CAD build for the part. Positions are in the model's coordinates, mm. Face numbers are marked on the shaded views. A direction names the side the tool comes from. Give positions to 0.01 mm unless a question says otherwise; leave off trailing zeros. Loops run counter-clockwise (first coordinate to the right, second up) from the corner with the lowest first, then second, coordinate; pieces in that order, holes last.
Item 1: Which spindle directions (+Z, -Z, +X, -X, +Y, -Y) get a long thin tool onto all of the face, cutting with end or side? Do the marked faces 5, 6 and 7. Say none if no direction does.
Item 2: Probe probe 1 along Z at (x, y) = (13.5, 10); probe 2 along Y at (x, z) = (0, 13.75); probe 3 along Y at (x, z) = (-5, 4.5) (3 decimals). List the from-to ranges inside material, lowest first.
Item 3: Saw through at A-A on y = 0. Give the cut face in (x, z), plus the area to 3 significant figures.
Item 4: Mould opens along X. For the marked faces 1, 2, 3 and 4 say: released by +X, released by -X, zero draft, split by the parting line, or undercut.
Item 5: Saw through at C-C on z = 5.25. Give the cut face in (x, y).
Item 6: Drop flat-ended pins along their axis: P1, Ø1.5, axis at y = -2.5, z = 13, coming from the -X side; P2, Ø4.5, axis at x = -15, y = -7, coming from the +Z side; P3, Ø8, axis at y = 3.5, z = 4.5, coming from the +X side. Give the stop position or say it passes through.
Item 7: Saw through at B-B on x = 0. Give the cut face in (y, z).
Item 8: Saw through at D-D on y = -15. Give the cut face in (x, z), plus the area to 3 significant figures.
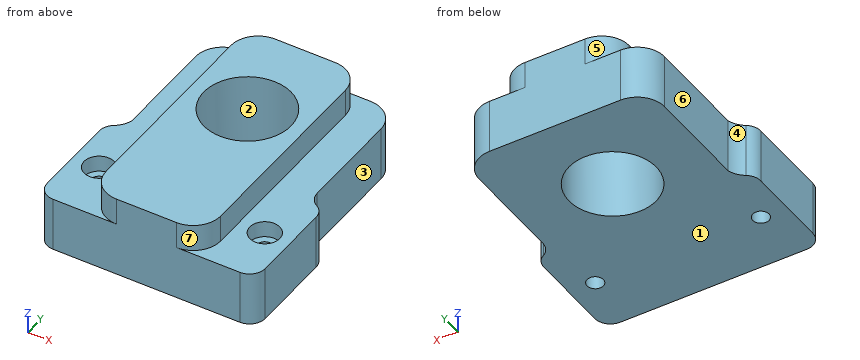
from build123d import *

# Parameters (mm, degrees)
F1_DEPTH  = 10
F3_DEPTH  = 5
F4_R      = 8
F5_DEPTH  = 25
F6_R      = 2.75
F6_R_2    = 1.5
F7_DEPTH  = 3
F8_DEPTH  = 25
F9_R      = 2.75
F9_R_2    = 1.5
F10_DEPTH = 3
F11_DEPTH = 25


with BuildPart() as f1:
    # F0 (on Top) → F1 (new body)
    with BuildSketch(Plane.XY):
        with BuildLine():
            Line((-17.1261427557, -29.75), (17.1261427557, -29.75))
            ThreePointArc((17.1261427557, -29.75), (19.1582667013, -28.9082667013), (20, -26.8761427557))
            Line((20, -26.8761427557), (20, -11.87280621))
            ThreePointArc((20, -11.87280621), (19.6060520694, -10.4205303214), (18.5322129268, -9.3664099655))
            ThreePointArc((18.5322129268, -9.3664099655), (17.4112395611, -8.2660209069), (17, -6.75))
            Line((17, -6.75), (17, 12))
            ThreePointArc((17, 12), (15.5355339059, 15.5355339059), (12, 17))
            Line((12, 17), (-12, 17))
            ThreePointArc((-12, 17), (-15.5355339059, 15.5355339059), (-17, 12))
            Line((-17, 12), (-17, -6.75))
            ThreePointArc((-17, -6.75), (-17.6456554571, -8.1178497679), (-18.730129695, -9.1722688421))
            ThreePointArc((-18.730129695, -9.1722688421), (-19.6627433299, -10.206041959), (-20, -11.5568613354))
            Line((-20, -11.5568613354), (-20, -26.8761427557))
            ThreePointArc((-20, -26.8761427557), (-19.1582667013, -28.9082667013), (-17.1261427557, -29.75))
        make_face()
    extrude(amount=F1_DEPTH)

    # F2 (on face) → F3 (join)
    with BuildSketch(Plane.XY.offset(10)):
        with BuildLine():
            Line((-10.5, 12), (-10.5, -24.75))
            ThreePointArc((-10.5, -24.75), (-9.0355339059, -28.2855339059), (-5.5, -29.75))
            Line((-5.5, -29.75), (5.5, -29.75))
            ThreePointArc((5.5, -29.75), (9.0355339059, -28.2855339059), (10.5, -24.75))
            Line((10.5, -24.75), (10.5, 12))
            ThreePointArc((10.5, 12), (9.0355339059, 15.5355339059), (5.5, 17))
            Line((5.5, 17), (-5.5, 17))
            ThreePointArc((-5.5, 17), (-9.0355339059, 15.5355339059), (-10.5, 12))
        make_face()
    extrude(amount=F3_DEPTH)

    # F4 (on face) → F5 (cut)
    with BuildSketch(Plane.XY.offset(15)):
        Circle(F4_R)
    extrude(amount=-F5_DEPTH, mode=Mode.SUBTRACT)

    # F6 (on face) → F7 (cut)
    with BuildSketch(Plane.XY.offset(10)):
        with Locations((-15.25, -19.2165020456)):
            Circle(F6_R)
        with Locations((-15.25, -19.2165020456)):
            Circle(F6_R_2, mode=Mode.SUBTRACT)
    extrude(amount=-F7_DEPTH, mode=Mode.SUBTRACT)

    # F8 (cut): a face of the model
    f8_faces = [f1.faces().sort_by_distance(p)[0] for p in [
        (-15.25, -19.2165020456, 10),
    ]]
    extrude(f8_faces, amount=-F8_DEPTH, mode=Mode.SUBTRACT)

    # F9 (on face) → F10 (cut)
    with BuildSketch(Plane.XY.offset(10)):
        with Locations((15.25, -19.3744744829)):
            Circle(F9_R)
        with Locations((15.25, -19.3744744829)):
            Circle(F9_R_2, mode=Mode.SUBTRACT)
    extrude(amount=-F10_DEPTH, mode=Mode.SUBTRACT)

    # F11 (cut): a face of the model
    f11_faces = [f1.faces().sort_by_distance(p)[0] for p in [
        (15.25, -19.3744744829, 10),
    ]]
    extrude(f11_faces, amount=-F11_DEPTH, mode=Mode.SUBTRACT)


solid = f1.part
Results below:
1. face 5: +Z, -X, +Y
1. face 6: +Z, -Z, -X, +Y
1. face 7: +Z, +X, -Y
2. probe 1: z = 0 to 10
2. probe 2: y = -29.75 to -8, 8 to 17
2. probe 3: y = -29.75 to -6.245, 6.245 to 17
3. outline: (-17, 0) - (-8, 0) - (-8, 15) - (-10.5, 15) - (-10.5, 10) - (-17, 10) - close; (8, 0) - (17, 0) - (17, 10) - (10.5, 10) - (10.5, 15) - (8, 15) - close
3. area: 205 mm2
4. face 1: zero draft
4. face 2: undercut
4. face 3: released by +X
4. face 4: released by -X
5. outline: (-20, -26.88) arc R2.87 ccw to (-17.13, -29.75) - (17.13, -29.75) arc R2.87 ccw to (20, -26.88) - (20, -11.87) arc R2.87 ccw to (18.53, -9.37) arc R3 cw to (17, -6.75) - (17, 12) arc R5 ccw to (12, 17) - (-12, 17) arc R5 ccw to (-17, 12) - (-17, -6.75) arc R4.24 cw to (-18.73, -9.17) arc R2.87 ccw to (-20, -11.56) - close; hole circle Ø3 at (-15.25, -19.22); hole circle Ø16 at (0, 0); hole circle Ø3 at (15.25, -19.37)
6. P1: stops at x = -10.5
6. P2: stops at z = 10
6. P3: stops at x = 17
7. outline: (-29.75, 0) - (-8, 0) - (-8, 15) - (-29.75, 15) - close; (8, 0) - (17, 0) - (17, 15) - (8, 15) - close
8. outline: (-20, 0) - (20, 0) - (20, 10) - (10.5, 10) - (10.5, 15) - (-10.5, 15) - (-10.5, 10) - (-20, 10) - close
8. area: 505 mm2
